```python
from build123d import *

# Parameters (mm, degrees)
F1_DEPTH = 5
F2_D     = 22


with BuildPart() as f1:
    # F0 (on Top) → F1 (new body)
    with BuildSketch(Plane.XY):
        with BuildLine():
            ThreePointArc((167.5, 0), (137.2079674184, 96.0740530888), (57.288374007, 157.3985139816))
            Line((57.288374007, 157.3985139816), (47.8828200656, 131.55696691))
            ThreePointArc((47.8828200656, 131.55696691), (114.6812862005, 80.3007010891), (140, 0))
            ThreePointArc((140, 0), (139.9786773219, -2.4433369012), (139.9147157827, -4.8859295383))
            Line((139.9147157827, -4.8859295384), (167.3979635257, -5.8456656977))
            ThreePointArc((167.3979635257, -5.8456656977), (167.4744889387, -2.9232780782), (167.5, 0))
        make_face()
        with BuildLine():
            ThreePointArc((194.8812112687, -6.805401857), (194.9703005555, -3.4032192553), (195, 0))
            ThreePointArc((195, 0), (159.7346486364, 111.8474050885), (66.6939279485, 183.2400610533))
            Line((66.6939279485, 183.2400610533), (57.288374007, 157.3985139816))
            ThreePointArc((57.288374007, 157.3985139816), (137.2079674184, 96.0740530888), (167.5, 0))
            ThreePointArc((167.5, 0), (167.4744889387, -2.9232780782), (167.3979635257, -5.8456656977))
            Line((167.3979635257, -5.8456656977), (194.8812112687, -6.805401857))
        make_face()
    extrude(amount=F1_DEPTH)

    # F2 (through all)
    with Locations(Plane(origin=(0, 0, 0), x_dir=(1, 0, 0), z_dir=(0, 0, -1))):
        with Locations((98.454029759, -135.5103465578), (159.3019664794, -51.7603465578), (159.3019664794, 51.7603465578)):
            Hole(F2_D / 2)


solid = f1.part
```
Part model, mm, in its own coordinate system. Coordinates: 2 decimals unless noted, no trailing zeros. Loops run counter-clockwise (first coordinate to the right, second up) from the corner with the lowest first, then second, coordinate; pieces in that order, holes last. Notation, with made-up numbers: (-22.75, 7) - (-9.75, 7) arc R31 cw to (-9.75, 40) - close; hole circle Ø2 at (88, 59). An arc over 180 degrees is marked (long way). Write item = value, one per line. Start each with the question number.
Item 1: Cut at A-A, the plane x = 92.5. Give the cut face in (y, z).
Item 2: Wall check: L1, parallel to Y at x = 159, z = 2; L2, parallel to Y at x = 97.5, z = 2.6; L3, parallel to X at y = 141.5, z = 4.7. Give the ranges that are in metal, low to high. Write a range as from..to.
Item 3: Cut at B-B, the plane y = 49.5. Give the cut face in (x, z), and give its area (3 significant figures).
Item 4: Flat gauge pins, fed straight in: pin 1 Ø1 at (y, z) = (127, 1) entering from +X; pin 2 Ø12 at (x, y) = (66, 118) entering from -Z; pin 3 Ø1.5 at (y, z) = (22.5, 4) entering from -X. Where does each tip first touch, or does it go through?
Item 5: Cut at C-C, the plane z = 1.6. Give the cut face in (x, y).
Item 6: Mould opens along Y. For faces 1 (the flat face through (137, 90, 5)), 2 (the cylindrical face through (149.14, 55.97, 2.53)), 3 (the cylindrical face through (87.96, 132.21, 2.53)) say: released by +Y, released by -Y, zero draft, split by the parting line, or undercut.
Item 7: Cut at D-D, the plane x = 125. Give the cut face in (y, z), and give its area (3 significant figures).
The answers:
q1.outline = (105.09, 0) - (126.26, 0) - (126.26, 5) - (105.09, 5) - close; (144.76, 0) - (171.66, 0) - (171.66, 5) - (144.76, 5) - close
q2.L1 = -5.55..40.76, 62.76..112.89
q2.L2 = 100.47..124.55, 146.47..168.87
q2.L3 = 51.5..89.23, 107.68..134.17
q3.outline = (130.96, 0) - (148.54, 0) - (148.54, 5) - (130.96, 5) - close; (170.07, 0) - (188.61, 0) - (188.61, 5) - (170.07, 5) - close
q3.area = 181 mm2
q4.pin_1 = 148.4
q4.pin_2 = 0
q4.pin_3 = 138.06
q5.outline = (47.88, 131.56) arc R140 cw to (139.91, -4.89) - (194.88, -6.81) arc R195 ccw to (66.69, 183.24) - close; hole circle Ø22 at (98.45, 135.51); hole circle Ø22 at (159.3, 51.76)
q6.face_1 = zero draft
q6.face_2 = undercut
q6.face_3 = undercut
q7.outline = (63.05, 0) - (149.67, 0) - (149.67, 5) - (63.05, 5) - close
q7.area = 433 mm2
